Autodesk Inventor part; units mm, degrees
ref_plane "YZ Plane" through (0, 0, 0) normal (1, 0, 0) x (0, 1, 0)
ref_plane "XZ Plane" through (0, 0, 0) normal (0, 1, 0) x (-1, 0, 0)
ref_plane "XY Plane" through (0, 0, 0) normal (0, 0, 1) x (1, 0, 0)
sketch "スケッチ1" plane through (0, 0, 0) normal (1, 0, 0) x (0, 1, 0)
  line L0 (0, 0) -> (15, 0)
  line L1 (15, 0) -> (15, -53)
  line L2 (15, -53) -> (0, -53)
  line L3 (0, -53) -> (0, 0)
  line L4 (9, -53) -> (-62.5, -53)
  line L5 (-62.5, -53) -> (-62.5, -59)
  line L6 (-62.5, -59) -> (9, -59)
  line L7 (9, -59) -> (9, -53)
  line L8 (15, -53) -> (9, -59)
  line L9 (0, -53) -> (0, -53)
  line L10 (10.5, -3) -> (4.5, -3)
  line L11 (4.5, -3) -> (4.5, -48)
  line L12 (4.5, -48) -> (10.5, -48)
  line L13 (10.5, -48) -> (10.5, -3)
  line L14 (15, -50.5) -> (0, -50.5)
  point P0 (7.5, 0)
  point P1 (7.5, -3)
  point P2 (-53.5, -56)
  point P3 (-59.5, -56)
  point P4 (-62.5, -56)
  dimension "d0" = 53
  dimension "d4" = 6
  dimension "d5" = 3
  dimension "d6" = 5
  dimension "d22" = 4.5
  dimension "d23" = 6
  dimension "d24" = 6
  dimension "d25" = 3
  dimension "d26" = 73
  dimension "d27" = 2.5
  dimension "d28" = 2.5
  dimension "d29" = 135
extrude "押し出し1" add sketch "スケッチ1" along normal blind 2 contours L0 L1 L14 L3 | L14 L1 L2 L3 | L2 L7 L6 L5 L4 | L8 L7 L2 | L13 L12 L11 L10
hole "穴1" at (0, 10.5, -3) at (0, 4.5, -3) at (0, 10.5, -48) at (0, 4.5, -48) at (0, -53.5, -56) at (0, -59.5, -56) direction (1, 0, 0) diameter 3 depth 8.8
sketch "スケッチ2" plane through (2, 0, 0) normal (1, 0, 0) x (0, 0, -1)
  line L0 (9, 10.5) -> (42, 10.5)
  line L1 (44, 8.5) -> (44, 6.5)
  line L2 (42, 4.5) -> (9, 4.5)
  line L3 (7, 6.5) -> (7, 8.5)
  line L4 (0, 15) -> (0, 0)
  circle A0 centre (3, 10.5) radius 1.5
  circle A1 centre (48, 10.5) radius 1.5
  arc A2 (9, 10.5) -> (7, 8.5) centre (9, 8.5) ccw
  arc A3 (7, 6.5) -> (9, 4.5) centre (9, 6.5) ccw
  arc A4 (42, 4.5) -> (44, 6.5) centre (42, 6.5) ccw
  arc A5 (44, 8.5) -> (42, 10.5) centre (42, 8.5) ccw
  point P0 (44, 10.5)
  point P1 (7, 7.5)
  point P2 (0, 7.5)
  dimension "d16" = 4
  dimension "d17" = 4
  dimension "d18" = 2
extrude "押し出し2" cut sketch "スケッチ2" against normal blind 2 contours L0 A5 L1 A4 L2 A3 L3 A2
fillet "フィレット1" radius 2 1 edges at (1, 15, -53)
fillet "フィレット2" radius 2 2 edges at (1, 9, -59) (1, 0, -53)
equation "\"d1\" = 1"
properties part number "Plate_Support" material "アルミニウム 6061"
Can you work these out from the model? Positions are in its coordinate system, mm. A direction names the side the tool comes from. Coordinates: 2 decimals unless noted, no trailing zeros. Order: outer loops, then holes, each group sorted by start corner. A loop starts at its lowest first (then second) coordinate and runs counter-clockwise, first axis right, second up.
1. If we section it at D-D (z = -26.5): Please give me the cut outline in (x, y).
2. If we section it at A-A (x = 0.3): Please give me the cut outline in (y, z).
3. I need wall thicknesses on line 1 (Y direction, x = 0.6, z = -48); line 2 (Y direction, x = 0.7, z = -56); line 3 (Y direction, x = 0.3, z = -38). Which ranges of each line are inside material? Lowest first, please.
4. For faces 5 (the face through (2, 2, -38)), 6 (the face through (1.01, 5.07, -43.4)), which set-ups out of +Z, -Z, +X, -X, +Y, -Y let a thin tool reach every point of the face, with its end or its side?
5. If we section it at C-C (y = -59.5): Please give me the cut outline in (x, z).
6. If we section it at B-B (z = -48): Please give me the cut outline in (x, y).
7. I'm going to push a flat-ended pin straight in: pin 1 (1 mm diameter, centred on x = 1, y = -35.5, fed in from +Z). Where does the tip first touch, or does it pass through?
8. Thinking about a two-plate mould opening in Z: for faces 1 (the face through (1.01, 4.05, -1.57)), 2 (the face through (1, 7, 0)), 3 (the face through (1, -28, -59)), 4 (the face through (1, 15, -26)), which applies, +Z half, -Z half, draft (parallel to the pull), parting line (faces both ways), or undercut?
Entries:
1. outline: (0, 0) - (2, 0) - (2, 4.5) - (0, 4.5) - close; (0, 10.5) - (2, 10.5) - (2, 15) - (0, 15) - close
2. outline: (-62.5, -59) - (8.17, -59) arc R2 ccw to (9.59, -58.41) - (14.41, -53.59) arc R2 ccw to (15, -52.17) - (15, 0) - (0, 0) - (0, -51) arc R2 cw to (-2, -53) - (-62.5, -53) - close; hole circle Ø3 at (-59.5, -56); hole circle Ø3 at (-53.5, -56); hole circle Ø3 at (4.5, -48); hole circle Ø3 at (4.5, -3); hole (4.5, -42) arc R2 ccw to (6.5, -44) - (8.5, -44) arc R2 ccw to (10.5, -42) - (10.5, -9) arc R2 ccw to (8.5, -7) - (6.5, -7) arc R2 ccw to (4.5, -9) - close; hole circle Ø3 at (10.5, -48); hole circle Ø3 at (10.5, -3)
3. line 1: y = 0 to 3, 6 to 9, 12 to 15
3. line 2: y = -62.5 to -61, -58 to -55, -52 to 12
3. line 3: y = 0 to 4.5, 10.5 to 15
4. face 5: +Z, -Z, +X, +Y, -Y
4. face 6: +X, -X
5. outline: (0, -59) - (2, -59) - (2, -57.5) - (0, -57.5) - close; (0, -54.5) - (2, -54.5) - (2, -53) - (0, -53) - close
6. outline: (0, 0) - (2, 0) - (2, 3) - (0, 3) - close; (0, 6) - (2, 6) - (2, 9) - (0, 9) - close; (0, 12) - (2, 12) - (2, 15) - (0, 15) - close
7. pin 1: stops at z = -53
8. face 1: undercut
8. face 2: +Z half
8. face 3: -Z half
8. face 4: draft
